Verification items for the finished model (mm, model axes). Face numbers are marked on the shaded views. A direction names the side the tool comes from. Give positions to 0.01 mm unless a question says otherwise; leave off trailing zeros. Loops run counter-clockwise (first coordinate to the right, second up) from the corner with the lowest first, then second, coordinate; pieces in that order, holes last. Notation, with made-up numbers: (53, 70.25) - (60, 70.25) arc R36 ccw to (60, 107.25) - close; hole circle Ø2 at (86.25, -6). An arc over 180 degrees is marked (long way). Answer in a Markdown table with one row per item.
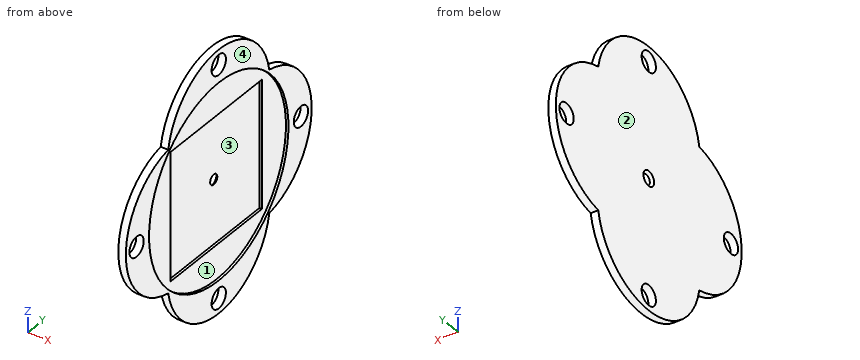
```python
from build123d import *

# Parameters (mm, degrees)
SKETCH2_R          = 2
BODY_DEPTH         = 0.75
SKETCH3_R          = 19.5
O_RING_SEAT_DEPTH  = 0.5
SKETCH11_W         = 25.5
SKETCH11_H         = 25.5
MESH_RECESS_DEPTH  = 0.5
SKETCH12_R         = 0.5
CUT_EXTRUDE4_DEPTH = 37.783148315
CHAMFER1_SIZE      = 1


with BuildPart() as part:
    # Sketch2 → Body (new, symmetric)
    with BuildSketch(Plane(origin=(0, 0, 0), x_dir=(0, 0, -1), z_dir=(1, 0, 0))):
        with BuildLine():
            ThreePointArc((-14.142135624, 14.142135624), (-26, 0), (-14.142135624, -14.142135624))
            ThreePointArc((-14.142135624, -14.142135624), (0, -26), (14.142135624, -14.142135624))
            ThreePointArc((14.142135624, -14.142135624), (26, 0), (14.142135624, 14.142135624))
            ThreePointArc((14.142135624, 14.142135624), (0, 26), (-14.142135624, 14.142135624))
        make_face()
        with Locations((0, 23)):
            Circle(SKETCH2_R, mode=Mode.SUBTRACT)
        with Locations((23, 0)):
            Circle(SKETCH2_R, mode=Mode.SUBTRACT)
        with Locations((0, -23)):
            Circle(SKETCH2_R, mode=Mode.SUBTRACT)
        with Locations((-23, 0)):
            Circle(SKETCH2_R, mode=Mode.SUBTRACT)
    extrude(amount=BODY_DEPTH, both=True)

    # Sketch3 → O-Ring Seat (cut)
    with BuildSketch(Plane(origin=(0.75, 0, 0), x_dir=(0, 0, -1), z_dir=(1, 0, 0))):
        Circle(SKETCH3_R)
    extrude(amount=-O_RING_SEAT_DEPTH, mode=Mode.SUBTRACT)

    # Sketch11 → Mesh Recess (cut)
    with BuildSketch(Plane(origin=(0.25, 0, 0), x_dir=(0, 0, -1), z_dir=(1, 0, 0))):
        Rectangle(SKETCH11_W, SKETCH11_H)
    extrude(amount=-MESH_RECESS_DEPTH, mode=Mode.SUBTRACT)

    # Sketch12 → Cut-Extrude4 (cut, through all)
    with BuildSketch(Plane(origin=(-0.25, 0, 0), x_dir=(0, 0, -1), z_dir=(1, 0, 0))):
        Circle(SKETCH12_R)
    extrude(amount=-CUT_EXTRUDE4_DEPTH, mode=Mode.SUBTRACT)

    # Chamfer1
    # the kernel refuses this chamfer: 1 mm, written as the material it takes off along each edge
    with BuildSketch(Plane(origin=(-0.75, 0, 0), x_dir=(0, 0, -1), z_dir=(0, -1, 0))) as chamfer1_piece_1:
        Polygon((0.5 + CHAMFER1_SIZE, 0), (0.5, CHAMFER1_SIZE), (0.5, 0), align=None)
    revolve(axis=Axis((-0.75, 0, 0), (1, 0, 0)), mode=Mode.SUBTRACT)


solid = part.part
```
Q1. Tool access check on the marked faces 3 and 4. Record the directions out of +Z, -Z, +X, -X, +Y, -Y that give a thin tool (end or side, any length) a straight path to the whole face; none if there is none.
Completed:
| item | result |
|---|---|
| face 3 | +X |
| face 4 | +Z, -Z, +X, +Y, -Y |
Q2. Go/stop test with a flat-tipped pin: P1, Ø10, axis at y = 11.5, z = -1.5, coming from the +X side. Record where the tip stops, or that it passes through.
Completed:
| item | result |
|---|---|
| P1 | x = 0.25 |
Q3. Sectioned sample at B-B (x = 0). Record the cut outline in (y, z).
Completed:
| item | result |
|---|---|
| outline | (-14.14, -14.14) arc R14.36 ccw to (14.14, -14.14) arc R14.36 ccw to (14.14, 14.14) arc R14.36 ccw to (-14.14, 14.14) arc R14.36 ccw to start; hole circle Ø4 at (-23, 0); hole (-12.75, -12.75) - (12.75, -12.75) - (12.75, 12.75) - (-12.75, 12.75) - close; hole circle Ø4 at (0, -23); hole circle Ø4 at (0, 23); hole circle Ø4 at (23, 0) |
Q4. Sectioned sample at D-D (z = -23). Record the cut outline in (x, y).
Completed:
| item | result |
|---|---|
| outline | (-0.75, -8.78) - (0.75, -8.78) - (0.75, -2) - (-0.75, -2) - close; (-0.75, 2) - (0.75, 2) - (0.75, 8.78) - (-0.75, 8.78) - close |
Q5. Thickness scan on line 1 (X direction, y = 14.5, z = 2.5); line 2 (Y direction, x = -0.05, z = -22.5); line 3 (X direction, y = 10, z = 10.5). Record the ranges inside material, lowest first.
Completed:
| item | result |
|---|---|
| line 1 | -0.75 to 0.25 |
| line 2 | -9.4 to -1.94, 1.94 to 9.4 |
| line 3 | -0.75 to -0.25 |
Q6. Sectioned sample at A-A (z = 0). Record the cut outline in (x, y).
Completed:
| item | result |
|---|---|
| outline | (-0.75, -26) - (0.75, -26) - (0.75, -25) - (-0.75, -25) - close; (-0.75, -21) - (0.75, -21) - (0.75, -19.5) - (0.25, -19.5) - (0.25, -12.75) - (-0.25, -12.75) - (-0.25, -1) - (-0.75, -1.5) - close; (-0.75, 1.5) - (-0.25, 1) - (-0.25, 12.75) - (0.25, 12.75) - (0.25, 19.5) - (0.75, 19.5) - (0.75, 21) - (-0.75, 21) - close; (-0.75, 25) - (0.75, 25) - (0.75, 26) - (-0.75, 26) - close |
Q7. Draft check along Z on the marked faces 1 and 2. Enter one of: +Z half, -Z half, draft (parallel to the pull), parting line (faces both ways), or undercut.
Completed:
| item | result |
|---|---|
| face 1 | undercut |
| face 2 | draft |
